Input: part model. Units: mm. Frame: model coordinates. Face numbers are marked on the shaded views. A direction names the side the tool comes from. Give positions to 0.01 mm unless a question says otherwise; leave off trailing zeros. Loops run counter-clockwise (first coordinate to the right, second up) from the corner with the lowest first, then second, coordinate; pieces in that order, holes last. Notation, with made-up numbers: M 38.25,51.25 L 96.25,51.25 A23 ccw 96.25,73.25 Z; hole C 46.5,44.5 d8. An arc over 180 degrees is marked long. Return JSON: item names as keys, results as strings. Group by question number.
Autodesk Inventor part; units mm, degrees
ref_plane "YZ Plane" through (0, 0, 0) normal (1, 0, 0) x (0, 1, 0)
ref_plane "XZ Plane" through (0, 0, 0) normal (0, 1, 0) x (-1, 0, 0)
ref_plane "XY Plane" through (0, 0, 0) normal (0, 0, 1) x (1, 0, 0)
sketch "Sketch1" plane through (0, 0, 0) normal (0, 1, 0) x (-1, 0, 0)
  line L0 (0, 0) -> (30, 0)
  line L1 (30, 0) -> (30, -44)
  line L2 (30, -44) -> (0, -44)
  line L3 (0, -44) -> (0, 0)
  circle A0 centre (24.9, -3.9) radius 1.5
  circle A1 centre (3.9, -3.9) radius 1.5
  circle A2 centre (3.9, -40.1) radius 1.5
  circle A3 centre (24.9, -40.1) radius 1.5
  circle A4 centre (15, -22) radius 9
  dimension "d0" = 44
  dimension "d1" = 30
  dimension "d2" = 3
  dimension "d3" = 3
  dimension "d4" = 3
  dimension "d5" = 3
  dimension "d8" = 3.9
  dimension "d9" = 3.9
  dimension "d10" = 3.9
  dimension "d11" = 3.9
  dimension "d12" = 3.9
  dimension "d14" = 21
  dimension "d15" = 3.9
  dimension "d17" = 21
  dimension "d18" = 18
  dimension "d19" = 22
  dimension "d20" = 15
extrude "Extrusion1" add sketch "Sketch1" along normal blind 5
sketch "Sketch2" plane through (0, 0, 0) normal (0, -1, 0) x (1, 0, 0)
  line L0 (-7.5, -44) -> (-22.5, -44)
  line L1 (-22.5, -44) -> (-22.5, -4)
  line L2 (-22.5, -4) -> (-7.5, -4)
  line L3 (-7.5, -4) -> (-7.5, -44)
  line L4 (0, 0) -> (-30, 0)
  line L5 (-30, -44) -> (0, -44)
  line L6 (0, -44) -> (0, 0)
  line L7 (-30, 0) -> (-30, -44)
  dimension "d24" = 4
  dimension "d25" = 0
  dimension "d26" = 15
  dimension "d27" = 7.5
  dimension "d28" = 7.5
extrude "Extrusion2" cut sketch "Sketch2" against normal blind 3 contours L0 L1 L2 L3
fillet "Fillet1" radius 2 4 edges at (0, 2.5, 0) (-30, 2.5, 0) (-30, 2.5, -44) (0, 2.5, -44)
sketch "Sketch3" plane through (0, 5, 0) normal (0, 1, 0) x (1, 0, 0)
  line L0 (-26, 23) -> (-4, 23)
  line L1 (-4, 23) -> (-4, 21)
  line L2 (-4, 21) -> (-26, 21)
  line L3 (-26, 21) -> (-26, 23)
  line L4 (-2, 44) -> (-28, 44)
  circle A0 centre (-15, 22) radius 9
  line L5 (-16, 33) -> (-14, 33)
  line L6 (-14, 33) -> (-14, 11)
  line L7 (-14, 11) -> (-16, 11)
  line L8 (-16, 11) -> (-16, 33)
  line L9 (-30, 42) -> (-30, 2)
  point P0 (0, 0)
  dimension "d32" = 2
  dimension "d33" = 21
  dimension "d34" = 11
  dimension "d35" = 11
  dimension "d36" = 14
  dimension "d37" = 2
  dimension "d38" = 11
  dimension "d39" = 11
extrude "Extrusion3" add sketch "Sketch3" along normal blind 40 contours L0 A0 L2 L3 | L0 L8 L2 A0 | L8 A0 L6 L0 | L0 L6 L2 L8 | L8 L5 L6 A0 | L0 A0 L2 L6 | L2 L6 A0 L8 | A0 L6 L7 L8 | L0 L1 L2 A0
sketch "Sketch4" plane through (-14, 5, -13.0557) normal (1, 0, 0) x (0, 0, -1)
  point P0 (-13.0557, -5)
properties part number "drzakfotorezistoru"
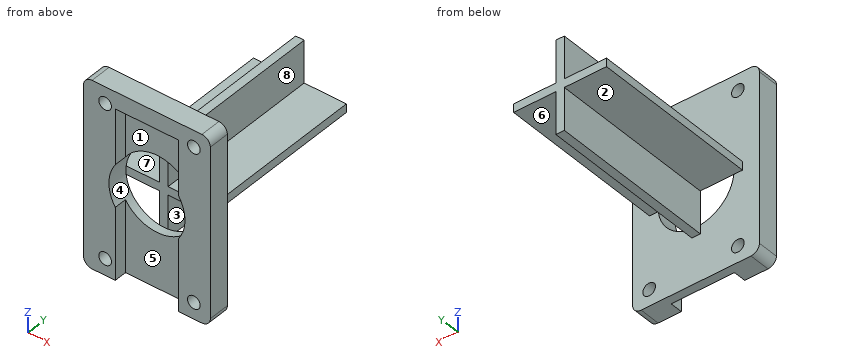
Item 1: Section B-B, the plane x = -24.9. Return loops of the section in (y, z), then the cut area to 3 significant figures.
Item 2: Material intervals for line 1 (Z direction, x = -3.9, y = 2.3); line 2 (Z direction, x = -16.75, y = 14); line 3 (X direction, y = 35.5, z = -19), sorted ascending. Write a range as from..to.
Item 3: Section C-C, the plane x = -15. Return loops of the section in (y, z).
Item 4: Pull-direction query (X, two-part tool) for the marked faces 1, 2 and 3; classes: pulls with the +X half, pulls with the -X half, needs draft (parallel to the pull), parting line crosses it, or undercut.
Item 5: Reachability of the marked faces 4, 5, 6, 7 and 8 from +Z, -Z, +X, -X, +Y, -Y: full face, straight path, thin tool, end or side. Return the list, or none.
Item 6: Section A-A, the plane z = -40.1. Return loops of the section in (x, y).
Item 7: Section D-D, the plane y = 36. Return loops of the section in (x, z).
Item 8: First-contact query: pin 1 Ø1.5 at (y, z) = (6.5, -12) entering from -X; pin 2 Ø8 at (x, z) = (-6, -13) entering from +Y; pin 3 Ø14.5 at (x, z) = (-14.5, -8.5) entering from -Y; pin 4 Ø3 at (x, y) = (-19, 16.5) entering from -Z. Flat tips, straight axial feed; report the tip coordinate or a pass-through.
Answer below:
{
 "1": {"outline": "M 0,-44 L 5,-44 L 5,-41.6 L 0,-41.6 Z; M 0,-38.6 L 5,-38.6 L 5,-23 L 45,-23 L 45,-21 L 5,-21 L 5,-5.4 L 0,-5.4 Z; M 0,-2.4 L 5,-2.4 L 5,0 L 0,0 Z", "area": "270 mm^2"},
 "2": {"line 1": "-44..-41.6, -38.6..-5.4, -2.4..0", "line 2": "-23..-21", "line 3": "-16..-14"},
 "3": {"outline": "M 0,-4 L 3,-4 L 3,-13 L 5,-13 L 5,-31 L 3,-31 L 3,-44 L 5,-44 L 5,-33 L 45,-33 L 45,-11 L 5,-11 L 5,0 L 0,0 Z"},
 "4": {"face 1": "undercut", "face 2": "needs draft", "face 3": "pulls with the +X half"},
 "5": {"face 4": "-Y", "face 5": "-Z, -Y", "face 6": "-Z, +X, +Y", "face 7": "+Z, -X, +Y", "face 8": "+Z, +X, +Y"},
 "6": {"outline": "M -30,0 L -26.4,0 L -26.4,5 L -30,5 Z; M -23.4,0 L -22.5,0 L -22.5,3 L -7.5,3 L -7.5,0 L -5.4,0 L -5.4,5 L -23.4,5 Z; M -2.4,0 L 0,0 L 0,5 L -2.4,5 Z"},
 "7": {"outline": "M -26,-23 L -16,-23 L -16,-33 L -14,-33 L -14,-23 L -4,-23 L -4,-21 L -14,-21 L -14,-11 L -16,-11 L -16,-21 L -26,-21 Z"},
 "8": {"pin 1": "x = -16", "pin 2": "y = 5", "pin 3": "y = 0", "pin 4": "z = -23"}
}
